Source: CAD feature listing. Evaluate the final solid. Frame: model axes, mm. Round coordinates to 2 decimals unless told otherwise and drop trailing zeros. Loops run counter-clockwise (first coordinate to the right, second up) from the corner with the lowest first, then second, coordinate; pieces in that order, holes last. Notation, with made-up numbers: (9.5, 45.25) -> (65.5, 45.25) arc R25 cw to (65.5, 70.25) -> close; hole circle Ø8 at (56, 70). An arc over 180 degrees is marked (long way). Put each result on its own line as item: value. Start each with the question number.
1. Cut plane C-C (x = -22). Return the cut outline in (y, z).
2. Draft query along X for faces 1 (the cylindrical face through (-4.88, -0.03, -1.08)), 2 (the flat face through (18.919, 0.028, 19.264)), 3 (the flat face through (6, 2, 0)). Return one class per face: pulls with the +X half, pulls with the -X half, needs draft (parallel to the pull), parting line crosses it, or undercut.
3. Cut plane A-A (y = 0.35). State how many separate pieces and enclosed holes the cut face has, then the cut area to 3 significant figures.
4. Cut plane B-B (z = -8). Return the cut outline in (x, y), then the cut area to 3 significant figures.
5. Cut plane D-D (z = 0). Return the cut outline in (x, y).
6. Material intervals for L1, parallel to Z at x = -0.5, y = 1.5; L2, parallel to X at y = 0.1, z = 0; L3, parallel to Z at x = 5.5, y = -0.1, sorted ascending.
7. Contact query for a flat-ended pin moving along its axis: pin 1 (1 mm diameter, centred on x = -14.5, y = 1.5, fed in from +Z). Output: stop coordinate, or through.
```python
from build123d import *

# Parameters (mm, degrees)
SKETCH1_R           = 1.5
SKETCH1_R_2         = 5
BOSS_EXTRUDE1_DEPTH = 2


with BuildPart() as part:
    # Sketch1 → Boss-Extrude1 (new, symmetric)
    with BuildSketch(Plane(origin=(0, 0, 0), x_dir=(1, 0, 0), z_dir=(0, 1, 0))):
        Polygon((11.27052257, 26.963900813), (-11.096894175, 27.035820049), (-26.963900813, 11.27052257), (-27.035820049, -11.096894175), (-11.27052257, -26.963900813), (11.096894175, -27.035820049), (26.963900813, -11.27052257), (27.035820049, 11.096894175), align=None)
        with Locations(Location((0, 22, 0), (0, 0, 270))):
            Circle(SKETCH1_R, mode=Mode.SUBTRACT)
        with Locations(Location((22, 0, 0), (0, 0, 270))):
            Circle(SKETCH1_R, mode=Mode.SUBTRACT)
        with Locations(Location((0, -22, 0), (0, 0, 270))):
            Circle(SKETCH1_R, mode=Mode.SUBTRACT)
        with Locations(Location((-22, 0, 0), (0, 0, 270))):
            Circle(SKETCH1_R, mode=Mode.SUBTRACT)
        with Locations(Location((0, 0, 0), (0, 0, 270))):
            Circle(SKETCH1_R_2, mode=Mode.SUBTRACT)
        with Locations(Location((-9.5, 0, 0), (0, 0, 270))):
            Circle(SKETCH1_R, mode=Mode.SUBTRACT)
        with Locations(Location((0, -8, 0), (0, 0, 270))):
            Circle(SKETCH1_R, mode=Mode.SUBTRACT)
        with Locations(Location((9.5, 0, 0), (0, 0, 270))):
            Circle(SKETCH1_R, mode=Mode.SUBTRACT)
        with Locations(Location((0, 8, 0), (0, 0, 270))):
            Circle(SKETCH1_R, mode=Mode.SUBTRACT)
    extrude(amount=BOSS_EXTRUDE1_DEPTH, both=True)


solid = part.part
```
Solution:
1. outline: (-2, -16.2) -> (2, -16.2) -> (2, -1.5) -> (-2, -1.5) -> close; (-2, 1.5) -> (2, 1.5) -> (2, 16.17) -> (-2, 16.17) -> close
2. face 1: undercut
2. face 2: pulls with the +X half
2. face 3: needs draft
3. separate pieces: 1
3. enclosed holes: 9
3. area: 2,280 mm^2
4. outline: (-26.97, -2) -> (-1.5, -2) -> (-1.5, 2) -> (-26.97, 2) -> close; (1.5, -2) -> (27.03, -2) -> (27.03, 2) -> (1.5, 2) -> close
4. area: 204 mm^2
5. outline: (-27, -2) -> (-23.5, -2) -> (-23.5, 2) -> (-27, 2) -> close; (-20.5, -2) -> (-11, -2) -> (-11, 2) -> (-20.5, 2) -> close; (-8, -2) -> (-5, -2) -> (-5, 2) -> (-8, 2) -> close; (5, -2) -> (8, -2) -> (8, 2) -> (5, 2) -> close; (11, -2) -> (20.5, -2) -> (20.5, 2) -> (11, 2) -> close; (23.5, -2) -> (27, -2) -> (27, 2) -> (23.5, 2) -> close
6. L1: z = -27 to -23.41, -20.59 to -9.41, -6.59 to -4.97, 4.97 to 6.59, 9.41 to 20.59, 23.41 to 27
6. L2: x = -27 to -23.5, -20.5 to -11, -8 to -5, 5 to 8, 11 to 20.5, 23.5 to 27
6. L3: z = -26.98 to 27.02
7. pin 1: stops at z = 24.22
